Check sheet for the modelled part. Datum: model origin and axes. Units: mm. A direction names the side the tool comes from. Give positions to 0.01 mm unless a question says otherwise; leave off trailing zeros. Write each loop counter-clockwise with the first axis right and the second up, starting at its lowest first coordinate (ties: lowest second). Pieces come first, ordered by that corner, then holes.
from build123d import *
from build123d.topology import SkipClean

# Parameters (mm, degrees)
TOP_SKETCH1_W                             = 34
TOP_SKETCH1_H                             = 37.5
TOP_SKETCH1_R                             = 1
TOP_SKETCH1_R_2                           = 2.5
BOSS_EXTRUDE4_DEPTH                       = 6
TOPRIGHTRISERBOSS_EXTRUDE5_START          = 14.4
TOPRIGHTRISER_R                           = 2.5
TOPRIGHTRISERBOSS_EXTRUDE5_DEPTH          = 14.4
TOPLEFTBOSS_EXTRUDE6_START                = 4.9
TOPLEFT_R                                 = 2.5
TOPLEFTBOSS_EXTRUDE6_DEPTH                = 4.9
MIDWALL_W                                 = 10.25
MIDWALL_H                                 = 3
MIDWALL_W_2                               = 4.5
MIDWALL_W_3                               = 3
MIDWALL_H_2                               = 37.5
MIDWALLBOSS_EXTRUDE7_DEPTH                = 28
BOTTOM_W                                  = 34
BOTTOM_H                                  = 37.5
BOTTOMBOSS_EXTRUDE8_DEPTH                 = 3
LOWERRIGHT_R                              = 2.5
LOWERRIGHTBOSS_EXTRUDE10_DEPTH            = 4.9
LOWERLEFT_R                               = 2.5
LOWERLEFTBOSS_EXTRUDE9_DEPTH              = 14.4
FILLET1_R                                 = 10
LINEARRAILMOUNTINGHOLES_SKETCH10_R        = 1
LINEARRAILMOUNTINGHOLESCUT_EXTRUDE1_DEPTH = 3
TOPRIGHTINSET_CUT_EXTRUDE1_DEPTH          = 1
TOPLEFTINSET_CUT_EXTRUDE2_DEPTH           = 1
LOWERLEFTINSET_CUT_EXTRUDE3_START         = -1
LOWERLEFTINSET_CUT_EXTRUDE3_DEPTH         = 1
LOWERRIGHTINSETCUT_EXTRUDE4_START         = -1
LOWERRIGHTINSETCUT_EXTRUDE4_DEPTH         = 1
PUSHPINHOLESKETCH1_R                      = 1
PUSHPINHOLECUT_EXTRUDE5_DEPTH             = 63.69968102


with BuildPart() as part:
    # Top-Sketch1 → Boss-Extrude4 (new body)
    with BuildSketch(Plane(origin=(0, 0, 0), x_dir=(1, 0, 0), z_dir=(0, 1, 0))):
        with Locations((17, 18.75)):
            Rectangle(TOP_SKETCH1_W, TOP_SKETCH1_H)
        with Locations(Location((8.5, 32.5, 0), (0, 0, 270))):
            Circle(TOP_SKETCH1_R, mode=Mode.SUBTRACT)
        with Locations(Location((8.5, 5, 0), (0, 0, 270))):
            Circle(TOP_SKETCH1_R, mode=Mode.SUBTRACT)
        with Locations(Location((8, 12.5, 0), (0, 0, 270))):
            Circle(TOP_SKETCH1_R_2, mode=Mode.SUBTRACT)
        with Locations(Location((20.5, 25, 0), (0, 0, 270))):
            Circle(TOP_SKETCH1_R_2, mode=Mode.SUBTRACT)
    extrude(amount=BOSS_EXTRUDE4_DEPTH)

    # TopRightRiser → TopRightRiserBoss-Extrude5 (add)
    with SkipClean():  # the faces are left unmerged after this step: merging them gives an invalid solid
        with BuildSketch(Plane.XZ.offset(TOPRIGHTRISERBOSS_EXTRUDE5_START)):
            with BuildLine():
                Line((5.75, -9.819048676), (5.75, 0))
                Line((5.75, 0), (10.25, 0))
                Line((10.25, 0), (10.25, -9.819048676))
                ThreePointArc((10.25, -9.819048676), (8, -16), (5.75, -9.819048676))
            make_face()
            with Locations(Location((8, -12.5, 0), (0, 0, 270))):
                Circle(TOPRIGHTRISER_R, mode=Mode.SUBTRACT)
        extrude(amount=-TOPRIGHTRISERBOSS_EXTRUDE5_DEPTH)

    # TopLeft → TopLeftBoss-Extrude6 (add)
    with SkipClean():  # the faces are left unmerged after this step: merging them gives an invalid solid
        with BuildSketch(Plane.XZ.offset(TOPLEFTBOSS_EXTRUDE6_START)):
            with BuildLine():
                Line((18.25, -22.319048676), (18.25, 0))
                Line((18.25, 0), (22.75, 0))
                Line((22.75, 0), (22.75, -22.319048676))
                ThreePointArc((22.75, -22.319048676), (20.5, -28.5), (18.25, -22.319048676))
            make_face()
            with Locations(Location((20.5, -25, 0), (0, 0, 270))):
                Circle(TOPLEFT_R, mode=Mode.SUBTRACT)
        extrude(amount=-TOPLEFTBOSS_EXTRUDE6_DEPTH)

    # MidWall → MidWallBoss-Extrude7 (add)
    with SkipClean():  # the faces are left unmerged after this step: merging them gives an invalid solid
        with BuildSketch(Plane(origin=(0, 0, 0), x_dir=(-1, 0, 0), z_dir=(0, -1, 0))):
            with Locations((-5.125, 1.5)):
                Rectangle(MIDWALL_W, MIDWALL_H)
            with Locations((-20.5, 1.5)):
                Rectangle(MIDWALL_W_2, MIDWALL_H)
            with Locations((-32.5, 18.75)):
                Rectangle(MIDWALL_W_3, MIDWALL_H_2)
        extrude(amount=MIDWALLBOSS_EXTRUDE7_DEPTH)

    # Bottom → BottomBoss-Extrude8 (add)
    with SkipClean():  # the faces are left unmerged after this step: merging them gives an invalid solid
        with BuildSketch(Plane.XZ.offset(28)):
            with Locations((17, -18.75)):
                Rectangle(BOTTOM_W, BOTTOM_H)
        extrude(amount=BOTTOMBOSS_EXTRUDE8_DEPTH)

    # LowerRight → LowerRightBoss-Extrude10 (add)
    with SkipClean():  # the faces are left unmerged after this step: merging them gives an invalid solid
        with BuildSketch(Plane(origin=(0, -28, 0), x_dir=(1, 0, 0), z_dir=(0, 1, 0))):
            with BuildLine():
                Line((5.75, 9.819048676), (5.75, 3))
                Line((5.75, 3), (10.25, 3))
                Line((10.25, 3), (10.25, 9.819048676))
                ThreePointArc((10.25, 9.819048676), (8, 16), (5.75, 9.819048676))
            make_face()
            with Locations(Location((8, 12.5, 0), (0, 0, 90))):
                Circle(LOWERRIGHT_R, mode=Mode.SUBTRACT)
        extrude(amount=LOWERRIGHTBOSS_EXTRUDE10_DEPTH)

    # LowerLeft → LowerLeftBoss-Extrude9 (add)
    with SkipClean():  # the faces are left unmerged after this step: merging them gives an invalid solid
        with BuildSketch(Plane(origin=(0, -28, 0), x_dir=(1, 0, 0), z_dir=(0, 1, 0))):
            with BuildLine():
                Line((18.25, 0), (22.75, 0))
                Line((22.75, 0), (22.75, 22.319048676))
                ThreePointArc((22.75, 22.319048676), (20.5, 28.5), (18.25, 22.319048676))
                Line((18.25, 22.319048676), (18.25, 0))
            make_face()
            with Locations(Location((20.5, 25, 0), (0, 0, 90))):
                Circle(LOWERLEFT_R, mode=Mode.SUBTRACT)
        extrude(amount=LOWERLEFTBOSS_EXTRUDE9_DEPTH)

    # Fillet1
    # the kernel refuses this fillet: 10 mm, written as the material it takes off along each edge
    with BuildSketch(Plane(origin=(0, 0, 0), x_dir=(1, 0, 0), z_dir=(0, -1, 0)), Plane(origin=(0, -28, 0), x_dir=(1, 0, 0), z_dir=(0, -1, 0))) as fillet1_piece_1:
        with BuildLine():
            CenterArc((FILLET1_R, -FILLET1_R), FILLET1_R, 90, 90)
            Line((0, -FILLET1_R), (0, 0))
            Line((0, 0), (FILLET1_R, 0))
        make_face()
    extrude(amount=28, mode=Mode.SUBTRACT)
    with BuildSketch(Plane(origin=(0, -3, -37.5), x_dir=(0, 0, 1), z_dir=(0, -1, 0))) as fillet1_piece_2:
        with BuildLine():
            CenterArc((FILLET1_R, -FILLET1_R), FILLET1_R, 90, 90)
            Line((0, -FILLET1_R), (0, 0))
            Line((0, 0), (FILLET1_R, 0))
        make_face()
    extrude(amount=53, mode=Mode.SUBTRACT)
    with BuildSketch(Plane(origin=(0, -25, -37.5), x_dir=(0, 0, 1), z_dir=(0, 1, 0))) as fillet1_piece_3:
        with BuildLine():
            CenterArc((FILLET1_R, FILLET1_R), FILLET1_R, 180, 90)
            Line((0, FILLET1_R), (0, 0))
            Line((0, 0), (FILLET1_R, 0))
        make_face()
    extrude(amount=56, mode=Mode.SUBTRACT)
    with BuildSketch(Plane(origin=(0, 0, 0), x_dir=(1, 0, 0), z_dir=(0, 1, 0))) as fillet1_piece_4:
        with BuildLine():
            CenterArc((FILLET1_R, FILLET1_R), FILLET1_R, 180, 90)
            Line((0, FILLET1_R), (0, 0))
            Line((0, 0), (FILLET1_R, 0))
        make_face()
    extrude(amount=31, mode=Mode.SUBTRACT)

    # LinearRailMountingHoles-Sketch10 → LinearRailMountingHolesCut-Extrude1 (cut)
    with BuildSketch(Plane(origin=(34, 0, 0), x_dir=(0, 0, -1), z_dir=(1, 0, 0))):
        with Locations((8.75, -2.5)):
            Circle(LINEARRAILMOUNTINGHOLES_SKETCH10_R)
        with Locations((8.75, -22.5)):
            Circle(LINEARRAILMOUNTINGHOLES_SKETCH10_R)
        with Locations((28.75, -22.5)):
            Circle(LINEARRAILMOUNTINGHOLES_SKETCH10_R)
        with Locations((28.75, -2.5)):
            Circle(LINEARRAILMOUNTINGHOLES_SKETCH10_R)
    extrude(amount=-LINEARRAILMOUNTINGHOLESCUT_EXTRUDE1_DEPTH, mode=Mode.SUBTRACT)

    # TopRightInset-Sketch1 → TopRightInset-Cut-Extrude1 (cut)
    with BuildSketch(Plane.XZ.offset(14.4)):
        with BuildLine():
            Line((5.75, -9.819048676), (5.75, -3))
            Line((5.75, -3), (10.25, -3))
            Line((10.25, -3), (10.25, -9.819048676))
            ThreePointArc((10.25, -9.819048676), (8, -9), (5.75, -9.819048676))
        make_face()
    extrude(amount=-TOPRIGHTINSET_CUT_EXTRUDE1_DEPTH, mode=Mode.SUBTRACT)

    # TopLeftInset-Sketch2 → TopLeftInset-Cut-Extrude2 (cut)
    with BuildSketch(Plane.XZ.offset(4.9)):
        with BuildLine():
            Line((18.25, -22.319048676), (18.25, -3))
            Line((18.25, -3), (22.75, -3))
            Line((22.75, -3), (22.75, -22.319048676))
            ThreePointArc((22.75, -22.319048676), (20.5, -21.5), (18.25, -22.319048676))
        make_face()
    extrude(amount=-TOPLEFTINSET_CUT_EXTRUDE2_DEPTH, mode=Mode.SUBTRACT)

    # LowerLeftInset-Sketch3 → LowerLeftInset-Cut-Extrude3 (cut)
    with BuildSketch(Plane(origin=(0, -13.6, 0), x_dir=(1, 0, 0), z_dir=(0, 1, 0)).offset(LOWERLEFTINSET_CUT_EXTRUDE3_START)):
        with BuildLine():
            Line((18.25, 22.319048676), (18.25, 3))
            Line((18.25, 3), (22.75, 3))
            Line((22.75, 3), (22.75, 22.319048676))
            ThreePointArc((22.75, 22.319048676), (20.5, 21.5), (18.25, 22.319048676))
        make_face()
    extrude(amount=LOWERLEFTINSET_CUT_EXTRUDE3_DEPTH, mode=Mode.SUBTRACT)

    # LowerRightInset-Sketch4 → LowerRightInsetCut-Extrude4 (cut)
    with BuildSketch(Plane(origin=(0, -23.1, 0), x_dir=(1, 0, 0), z_dir=(0, 1, 0)).offset(LOWERRIGHTINSETCUT_EXTRUDE4_START)):
        with BuildLine():
            Line((5.75, 9.819048676), (5.75, 3))
            Line((5.75, 3), (10.25, 3))
            Line((10.25, 3), (10.25, 9.819048676))
            ThreePointArc((10.25, 9.819048676), (8, 9), (5.75, 9.819048676))
        make_face()
    extrude(amount=LOWERRIGHTINSETCUT_EXTRUDE4_DEPTH, mode=Mode.SUBTRACT)

    # PushPinHoleSketch1 → PushPinHoleCut-Extrude5 (cut, through all)
    with BuildSketch(Plane.XZ.offset(31)):
        with Locations(Location((20.5, -25, 0), (0, 0, 270))):
            Circle(PUSHPINHOLESKETCH1_R)
        with Locations(Location((8, -12.5, 0), (0, 0, 270))):
            Circle(PUSHPINHOLESKETCH1_R)
    extrude(amount=-PUSHPINHOLECUT_EXTRUDE5_DEPTH, mode=Mode.SUBTRACT)


solid = part.part
1) Sectioned sample at C-C on y = -17. Record the boundary of the cut face in (x, z).
2) Draft check along Y on faces 4 (the flat face through (15, -28, -18)), 5 (the cylindrical face through (19, -21, -23)), 6 (the flat face through (17, -31, -18)), 7 (the flat face through (10.25, -11, -4)). Enter one of: +Y half, -Y half, draft (parallel to the pull), parting line (faces both ways), or undercut.
3) Gauge pin test, flat ends, axial feed: pin 1 (2.5 mm diameter, centred on y = -2.5, z = -8.75, fed in from -X); pin 2 (5.5 mm diameter, centred on x = 20.5, z = -25, fed in from +Y); pin 3 (3 mm diameter, centred on x = 12.5, y = -11, fed in from -Z); pin 4 (8 mm diameter, centred on x = 6.5, y = -12, fed in from -Z). Record the tip position at first contact, or that the pin passes through.
4) Sectioned sample at B-B on x = 20.5. Record the boundary of the cut face in (y, z).
5) Access from +Z, -Z, +X, -X, +Y, -Y to the whole of each face (thin tool, end or side, straight path). Record for faces 1 (the flat face through (22, -28, -25)), 2 (the flat face through (9, -14.4, -10)), 3 (the flat face through (5.75, -7, -6)).
6) Scan lines: L1, parallel to Y at x = 11, z = -22; L2, parallel to X at y = -26.3, z = -12.5; L3, parallel to Z at x = 8, y = -24. Record each from-to range of solid material in increasing order.
7) Sectioned sample at A-A on y = -26. Record the boundary of the cut face in (x, z).
8) Sectioned sample at D-D on z = -25. Record the boundary of the cut face in (x, y), then the cut area to 3 significant figures.
Answers below:
1. outline: (2.86, -3) - (10.25, -3) - (10.25, 0) - (10, 0) arc R10 ccw to start; (18.25, -22.32) arc R3.5 ccw (long way) to (22.75, -22.32) - (22.75, 0) - (18.25, 0) - close; (31, -37.5) - (34, -37.5) - (34, 0) - (31, 0) - close; hole circle Ø5 at (20.5, -25)
2. face 4: undercut
2. face 5: draft
2. face 6: -Y half
2. face 7: undercut
3. pin 1: stops at x = 5.55
3. pin 2: stops at y = 6
3. pin 3: stops at z = -14.3
3. pin 4: stops at z = -16
4. outline: (-31, -37.5) - (-28, -37.5) - (-28, -28.5) - (-13.6, -28.5) - (-13.6, -27.5) - (-28, -27.5) - (-28, -26) - (-31, -26) - close; (-31, -24) - (-28, -24) - (-28, -22.5) - (-13.6, -22.5) - (-13.6, -21.5) - (-14.6, -21.5) - (-14.6, -3) - (-3.9, -3) - (-3.9, -21.5) - (-4.9, -21.5) - (-4.9, -22.5) - (6, -22.5) - (6, 0) - (-31, 0) - close; (-4.9, -28.5) - (0, -28.5) - (0, -37.5) - (6, -37.5) - (6, -27.5) - (-4.9, -27.5) - close
5. face 1: +Y
5. face 2: -Z, -X
5. face 3: -X
6. L1: y = -31 to -28, 0 to 6
6. L2: x = 4.5 to 5.5, 10.5 to 11.5, 18.25 to 22.75, 31 to 34
6. L3: z = -16 to -15, -10 to -9, -3 to -0.2
7. outline: (2.86, -3) - (5.75, -3) - (5.75, -9.82) arc R3.5 ccw (long way) to (10.25, -9.82) - (10.25, 0) - (10, 0) arc R10 ccw to start; (18.25, -22.32) arc R3.5 ccw (long way) to (22.75, -22.32) - (22.75, 0) - (18.25, 0) - close; (31, -37.5) - (34, -37.5) - (34, 0) - (31, 0) - close; hole circle Ø5 at (8, -12.5); hole circle Ø5 at (20.5, -25)
8. outline: (0, -31) - (19.5, -31) - (19.5, -28) - (18, -28) - (18, -13.6) - (17, -13.6) - (17, -28) - (0, -28) - close; (0, 0) - (17, 0) - (17, -4.9) - (18, -4.9) - (18, 6) - (0, 6) - close; (21.5, -31) - (34, -31) - (34, 6) - (23, 6) - (23, -4.9) - (24, -4.9) - (24, 0) - (31, 0) - (31, -28) - (24, -28) - (24, -13.6) - (23, -13.6) - (23, -28) - (21.5, -28) - close
8. area: 393 mm2
